Part model, mm, in its own coordinate system. A direction names the side the tool comes from. Give positions to 0.01 mm unless a question says otherwise; leave off trailing zeros. Order: outer loops, then holes, each group sorted by start corner. A loop starts at its lowest first (then second) coordinate and runs counter-clockwise, first axis right, second up. Notation, with made-up numbers: (68, -26.5) - (103, -26.5) arc R3 ccw to (103, -22.5) - close; hole circle Ø3 at (42, 75). An arc over 180 degrees is marked (long way). One line per item, written item: value.
```python
from build123d import *

# Parameters (mm, degrees)
SKETCH1_W           = 28
SKETCH1_H           = 14.2
BOSS_EXTRUDE1_DEPTH = 33
SKETCH2_R           = 2.321908149
BOSS_EXTRUDE3_DEPTH = 4
SKETCH3_W           = 6.974752534
SKETCH3_H           = 3.176308394
BOSS_EXTRUDE4_DEPTH = 5
SKETCH4_W           = 5.77752576
SKETCH4_H           = 2.149777027
CUT_EXTRUDE1_DEPTH  = 5
SKETCH6_W           = 14.2
SKETCH6_H           = 2.892759627
BOSS_EXTRUDE5_DEPTH = 6
SKETCH11_W          = 14.2
SKETCH11_H          = 2.89
BOSS_EXTRUDE6_DEPTH = 6
SKETCH12_R          = 1.651
CUT_EXTRUDE4_DEPTH  = 6
SKETCH17_R          = 1.651
CUT_EXTRUDE5_DEPTH  = 45.435355427


with BuildPart() as part:
    # Sketch1 → Boss-Extrude1 (new body)
    with BuildSketch(Plane(origin=(0, 0, 0), x_dir=(1, 0, 0), z_dir=(0, 1, 0))):
        with Locations((-14, 7.1)):
            Rectangle(SKETCH1_W, SKETCH1_H)
    extrude(amount=BOSS_EXTRUDE1_DEPTH)

    # Sketch2 → Boss-Extrude3 (add)
    with BuildSketch(Plane(origin=(0, 33, 0), x_dir=(1, 0, 0), z_dir=(0, 1, 0))):
        with Locations(Location((-5.331542912, 7.506333926, 0), (0, 0, 270))):
            Circle(SKETCH2_R)
    extrude(amount=BOSS_EXTRUDE3_DEPTH)

    # Sketch3 → Boss-Extrude4 (add)
    with BuildSketch(Plane(origin=(0, 0, 0), x_dir=(0, 0, -1), z_dir=(1, 0, 0))):
        with Locations((7.1, 2.624490745)):
            Rectangle(SKETCH3_W, SKETCH3_H)
    extrude(amount=BOSS_EXTRUDE4_DEPTH)

    # Sketch4 → Cut-Extrude1 (cut)
    with BuildSketch(Plane(origin=(5, 0, 0), x_dir=(0, 0, -1), z_dir=(1, 0, 0))):
        with Locations((7.1, 2.467865933)):
            Rectangle(SKETCH4_W, SKETCH4_H)
    extrude(amount=-CUT_EXTRUDE1_DEPTH, mode=Mode.SUBTRACT)

    # Sketch6 → Boss-Extrude5 (add)
    with BuildSketch(Plane.ZY.offset(28)):
        with Locations((-7.1, 23.390302975)):
            Rectangle(SKETCH6_W, SKETCH6_H)
    extrude(amount=BOSS_EXTRUDE5_DEPTH)

    # Sketch11 → Boss-Extrude6 (add)
    with BuildSketch(Plane(origin=(0, 0, 0), x_dir=(0, 0, -1), z_dir=(1, 0, 0))):
        with Locations((7.1, 23.445)):
            Rectangle(SKETCH11_W, SKETCH11_H)
    extrude(amount=BOSS_EXTRUDE6_DEPTH)

    # Sketch12 → Cut-Extrude4 (cut)
    with BuildSketch(Plane(origin=(0, 24.89, 0), x_dir=(1, 0, 0), z_dir=(0, 1, 0))):
        with Locations(Location((3.594494482, 7.1, 0), (0, 0, 270))):
            Circle(SKETCH12_R)
    extrude(amount=-CUT_EXTRUDE4_DEPTH, mode=Mode.SUBTRACT)

    # Sketch17 → Cut-Extrude5 (cut, through all)
    with BuildSketch(Plane(origin=(0, 24.836682788, 0), x_dir=(1, 0, 0), z_dir=(0, 1, 0))):
        with Locations(Location((-31.335208853, 7.1, 0), (0, 0, 270))):
            Circle(SKETCH17_R)
    extrude(amount=-CUT_EXTRUDE5_DEPTH, mode=Mode.SUBTRACT)


solid = part.part
```
1) Mould opens along Z. For faces 5 (the flat face through (2, 3, -3.613)), 6 (the flat face through (0, 2, -7)), 7 (the flat face through (-28, 11, -7)) say: released by +Z, released by -Z, zero draft, split by the parting line, or undercut.
Outcome:
face 5: released by +Z
face 6: undercut
face 7: zero draft
2) Cut at D-D, the plane x = -1. Give the cut face in (y, z).
Outcome:
outline: (0, -14.2) - (33, -14.2) - (33, 0) - (0, 0) - close
3) Which spindle directions (+Z, -Z, +X, -X, +Y, -Y) get a long thin tool onto all of the face, cutting with end or side? Do faces 1 (the flat face through (-31, 21.944, -9)), 2 (the flat face through (-28, 29, -7)), 3 (the flat face through (2, 1.036, -7)), 4 (the flat face through (2, 4.213, -7)). Say none if no direction does.
Outcome:
face 1: +Z, -Z, -X, -Y
face 2: +Z, -Z, -X, +Y
face 3: +Z, -Z, +X, -Y
face 4: +Z, -Z, +X
4) Drill centre lines: line 1 along X through (y, z) = (23, -7.5); line 2 along Y through (x, z) = (-17, -4.75); line 3 along X through (y, z) = (2.5, -8.5). Where is each one in solid material? Low to high. Write a range as from..to.
Outcome:
line 1: x = -34..-32.94, -29.73..1.99, 5.2..6
line 2: y = 0..33
line 3: x = -28..0
5) Pin check, flat tips, straight feed: pin 1 (4.5 mm diameter, centred on y = 14, z = -9, fed in from -X); pin 2 (1.1 mm diameter, centred on x = 2.5, y = 2.5, fed in from -Z); pin 3 (2.5 mm diameter, centred on x = 2, z = -8, fed in from -Y); pin 4 (2.5 mm diameter, centred on x = -31.34, z = -7.1, fed in from -Y). Stop position of each tip, or through.
Outcome:
pin 1: stops at x = -28
pin 2: stops at z = -10.59
pin 3: stops at y = 1.04
pin 4: passes through
6) Cut at A-A, the plane z = -8. Give the number of separate pieces and of enclosed holes in the cut face, then the cut area to 3 significant figures.
Outcome:
separate pieces: 3
enclosed holes: 0
area: 966 mm^2
7) Cut at B-B, the plane z = -2. Give the cut face in (x, y), then the cut area to 3 significant figures.
Outcome:
outline: (-34, 21.94) - (-28, 21.94) - (-28, 0) - (0, 0) - (0, 22) - (6, 22) - (6, 24.89) - (0, 24.89) - (0, 33) - (-28, 33) - (-28, 24.84) - (-34, 24.84) - close
area: 959 mm^2
8) Cut at C-C, the plane y = 18. Give the cut face in (x, z), then the cut area to 3 significant figures.
Outcome:
outline: (-28, -14.2) - (0, -14.2) - (0, 0) - (-28, 0) - close
area: 398 mm^2
